```python
from build123d import *

# Parameters (mm, degrees)
F0_W      = 20
F0_H      = 46
F1_DEPTH  = 3
F2_W      = 20
F2_H      = 3
F3_DEPTH  = 13
F6_DEPTH  = 25
F7_DEPTH  = 25
F9_DEPTH  = 20
F11_DEPTH = 20
F12_DEPTH = 25
F13_DEPTH = 25
F14_W     = 5
F14_H     = 12
F15_DEPTH = 13
F17_DEPTH = 25
F18_R     = 0.5


# Not quite as in the source:
# - ends of sketch curves that miss each other by under 0.0002 mm in the source are joined


with BuildPart() as f1:
    # F0 (on Top) → F1 (new body)
    with BuildSketch(Plane.XY):
        with Locations((10, -23)):
            Rectangle(F0_W, F0_H)
    extrude(amount=F1_DEPTH)

    # F2 (on face) → F3 (join)
    with BuildSketch(Plane.XY.offset(3)):
        with Locations((10, -15.5)):
            Rectangle(F2_W, F2_H)
        with Locations((10, -30.5)):
            Rectangle(F2_W, F2_H)
    extrude(amount=F3_DEPTH)

    # F5 (on face) → F6 (cut)
    with BuildSketch(Plane.XY.offset(3)):
        with BuildLine():
            Line((10, -39), (8.5, -39))
            ThreePointArc((8.5, -39), (10, -40.5), (11.5, -39))
            ThreePointArc((11.5, -39), (11.0606601718, -37.9393398282), (10, -37.5))
            Line((10, -37.5), (10, -39))
        make_face()
        with BuildLine():
            ThreePointArc((10, -37.5), (8.9393398282, -37.9393398282), (8.5, -39))
            Line((8.5, -39), (10, -39))
            Line((10, -39), (10, -37.5))
        make_face()
    extrude(amount=-F6_DEPTH, mode=Mode.SUBTRACT)

    # F5 (on face) → F7 (cut)
    with BuildSketch(Plane.XY.offset(3)):
        with BuildLine():
            ThreePointArc((11.5000007078, -7), (11.0606608796, -5.9393398282), (10.0000007078, -5.5))
            Line((10.0000007078, -5.5), (10.0000007078, -7))
            Line((10.0000007078, -7), (10, -8.5))
            ThreePointArc((10, -8.5), (11.0606606293, -8.060660422), (11.5000007078, -7))
        make_face()
        with BuildLine():
            Line((10.0000007078, -7), (8.5000007078, -7))
            ThreePointArc((8.5000007078, -7), (8.9393402858, -8.0606599215), (10, -8.5))
            Line((10, -8.5), (10.0000007078, -7))
        make_face()
        with BuildLine():
            Line((10.0000007078, -7), (10.0000007078, -5.5))
            ThreePointArc((10.0000007078, -5.5), (8.939340536, -5.9393398282), (8.5000007078, -7))
            Line((8.5000007078, -7), (10.0000007078, -7))
        make_face()
    extrude(amount=-F7_DEPTH, mode=Mode.SUBTRACT)

    # F8 (on face) → F9 (join)
    with BuildSketch(Plane(origin=(0, 0, 0), x_dir=(0, -1, 0), z_dir=(-1, 0, 0))):
        Polygon((46, 3), (32, 16), (29, 16), (46, 0), align=None)
    extrude(amount=-F9_DEPTH)

    # F10 (on face) → F11 (join)
    with BuildSketch(Plane.YZ.offset(20)):
        Polygon((0, 3), (-14, 16), (-14, 13.1764705882), (-3.1875, 3), align=None)
    extrude(amount=-F11_DEPTH)

    # F5 (on face) → F12 (cut)
    with BuildSketch(Plane.XY.offset(3)):
        with BuildLine():
            Line((10, -39), (8.5, -39))
            ThreePointArc((8.5, -39), (10, -40.5), (11.5, -39))
            ThreePointArc((11.5, -39), (11.0606601718, -37.9393398282), (10, -37.5))
            Line((10, -37.5), (10, -39))
        make_face()
        with BuildLine():
            ThreePointArc((10, -37.5), (8.9393398282, -37.9393398282), (8.5, -39))
            Line((8.5, -39), (10, -39))
            Line((10, -39), (10, -37.5))
        make_face()
    extrude(amount=F12_DEPTH, mode=Mode.SUBTRACT)

    # F5 (on face) → F13 (cut)
    with BuildSketch(Plane.XY.offset(3)):
        with BuildLine():
            ThreePointArc((11.5000007078, -7), (11.0606608796, -5.9393398282), (10.0000007078, -5.5))
            Line((10.0000007078, -5.5), (10.0000007078, -7))
            Line((10.0000007078, -7), (10, -8.5))
            ThreePointArc((10, -8.5), (11.0606606293, -8.060660422), (11.5000007078, -7))
        make_face()
        with BuildLine():
            Line((10.0000007078, -7), (8.5000007078, -7))
            ThreePointArc((8.5000007078, -7), (8.9393402858, -8.0606599215), (10, -8.5))
            Line((10, -8.5), (10.0000007078, -7))
        make_face()
        with BuildLine():
            Line((10.0000007078, -7), (10.0000007078, -5.5))
            ThreePointArc((10.0000007078, -5.5), (8.939340536, -5.9393398282), (8.5000007078, -7))
            Line((8.5000007078, -7), (10.0000007078, -7))
        make_face()
    extrude(amount=F13_DEPTH, mode=Mode.SUBTRACT)

    # F14 (on face) → F15 (join)
    with BuildSketch(Plane.XY.offset(3)):
        with Locations((6.5, -23)):
            Rectangle(F14_W, F14_H)
    extrude(amount=F15_DEPTH)

    # F16 (on face) → F17 (cut)
    with BuildSketch(Plane(origin=(4, 0, 0), x_dir=(0, -1, 0), z_dir=(-1, 0, 0))):
        with BuildLine():
            Line((19.5, 16), (19.5, 9))
            ThreePointArc((19.5, 9), (23, 12.5), (26.5, 9))
            Line((26.5, 9), (26.5, 16))
            Line((26.5, 16), (19.5, 16))
        make_face()
        with BuildLine():
            ThreePointArc((26.5, 9), (23, 12.5), (19.5, 9))
            Line((19.5, 9), (23, 9))
            Line((23, 9), (26.5, 9))
        make_face()
        with BuildLine():
            ThreePointArc((19.5, 9), (20.5251262658, 6.5251262658), (23, 5.5))
            Line((23, 5.5), (23, 9))
            Line((23, 9), (19.5, 9))
        make_face()
        with BuildLine():
            Line((23, 9), (23, 5.5))
            ThreePointArc((23, 5.5), (25.4748737342, 6.5251262658), (26.5, 9))
            Line((26.5, 9), (23, 9))
        make_face()
    extrude(amount=-F17_DEPTH, mode=Mode.SUBTRACT)

    # F18
    f18_edges = [f1.edges().sort_by_distance(p)[0] for p in [
        (2, -17, 16),
        (2, -29, 16),
    ]]
    fillet(f18_edges, radius=F18_R)


solid = f1.part
```
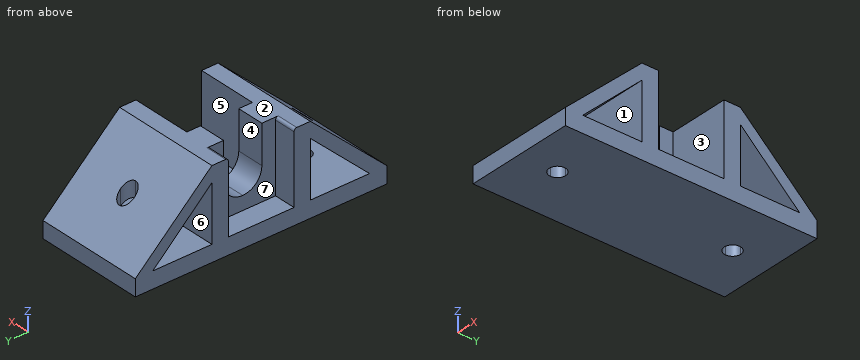
Geometry check sheet. Reference: the model listing, model coordinates, mm. Face numbers are marked on the shaded views. A direction names the side the tool comes from. Give positions to 0.01 mm unless a question says otherwise; leave off trailing zeros. Write each loop counter-clockwise with the first axis right and the second up, starting at its lowest first coordinate (ties: lowest second). Pieces come first, ordered by that corner, then holes.
1) Section check A-A, the plane z = 1.5. Record the boundary of the cut face in (x, y).
2) Section check D-D, the plane z = 14. Record the boundary of the cut face in (x, y), and give its area (3 significant figures).
3) Section check C-C, the plane x = 15.25. Record the boundary of the cut face in (y, z), and give its area (3 significant figures).
4) Access from +Z, -Z, +X, -X, +Y, -Y to the whole of each face (thin tool, end or side, straight path). Record for the marked faces 4, 5, 6 and 7.
5) Material ranges on L1, parallel to Y at x = 9.25, z = 9.25; L2, parallel to Y at x = 14.75, z = 3.5; L3, parallel to Y at x = 7.75, z = 3.5, recorded low to high.
6) Section check B-B, the plane y = -11.5. Record the boundary of the cut face in (x, z), and give its area (3 significant figures).
7) Release check for a two-part mould opening along Z. For the marked faces 1, 2 and 3 record: pulls with the +Z half, pulls with the -Z half, needs draft (parallel to the pull), parting line crosses it, or undercut.
8) Gauge pin test, flat ends, axial feed: pin 1 (8.5 mm diameter, centred on x = 9, y = -40, fed in from +Z); pin 2 (1 mm diameter, centred on x = 3, y = -11.5, fed in from -Z); pin 3 (5 mm diameter, centred on x = 5, z = 9, fed in from -Y); pin 4 (1.5 mm diameter, centred on x = 5.5, z = 11.5, fed in from +Y). Record the tip position at first contact, or that the pin passes through.
Computed:
1. outline: (0, -46) - (20, -46) - (20, 0) - (0, 0) - close; hole circle Ø3 at (10, -39); hole circle Ø3 at (10, -7)
2. outline: (0, -34.15) - (20, -34.15) - (20, -29) - (9, -29) - (9, -26.5) - (4, -26.5) - (4, -29) - (0, -29) - close; (0, -17) - (4, -17) - (4, -19.5) - (9, -19.5) - (9, -17) - (20, -17) - (20, -11.85) - (0, -11.85) - close
2. area: 231 mm2
3. outline: (-46, 0) - (0, 0) - (0, 3) - (-14, 16) - (-17, 16) - (-17, 3) - (-29, 3) - (-29, 16) - (-32, 16) - (-46, 3) - close; hole (-42.81, 3) - (-32, 3) - (-32, 13.18) - close; hole (-14, 3) - (-3.19, 3) - (-14, 13.18) - close
3. area: 288 mm2
4. face 4: +Z, +X, -X
4. face 5: +Z, +X
4. face 6: +X, -X
4. face 7: +Z, -X
5. L1: y = -37.7 to -36.17, -32 to -29, -17 to -14, -9.83 to -8.3
5. L2: y = -45.46 to -42.28, -32 to -29, -17 to -14, -3.72 to -0.54
5. L3: y = -45.46 to -42.28, -32 to -14, -3.72 to -0.54
6. outline: (0, 0) - (20, 0) - (20, 3) - (0, 3) - close; (0, 10.82) - (20, 10.82) - (20, 13.68) - (0, 13.68) - close
6. area: 117 mm2
7. face 1: undercut
7. face 2: pulls with the +Z half
7. face 3: needs draft
8. pin 1: stops at z = 12.52
8. pin 2: stops at z = 0
8. pin 3: stops at y = -42.23
8. pin 4: stops at y = -8.35
